The listing builds one solid part. Answer for the finished solid, in the listing's coordinates (mm). Face numbers are marked on the shaded views. A direction names the side the tool comes from. Round coordinates to 2 decimals unless told otherwise and drop trailing zeros. Order: outer loops, then holes, each group sorted by start corner. A loop starts at its lowest first (then second) coordinate and runs counter-clockwise, first axis right, second up. Notation, with made-up numbers: (18.5, 34.5) -> (57.5, 34.5) arc R19 cw to (57.5, 56.5) -> close; hole circle Ø3 at (8.25, 67). An arc over 180 degrees is marked (long way). Answer in a Markdown table with one row per item. Add a question column.
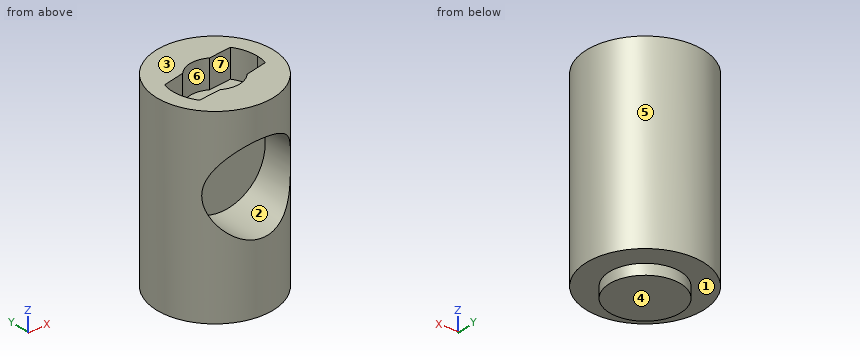
```python
from build123d import *

# Parameters (mm, degrees)
SKETCH_1_R          = 8.2
EXTRUDE_1_DEPTH     = 26.65
SKETCH_3_R          = 5
EXTRUDE_2_DEPTH     = 1.5
CUT_EXTRUDE_1_DEPTH = 4
CUT_EXTRUDE_START   = -1
SKETCH_5_R          = 6.25
CUT_EXTRUDE_2_DEPTH = 10


with BuildPart() as part:
    # Эскиз1 → Бобышка-Вытянуть1 (new body)
    with BuildSketch(Plane.XY):
        Circle(SKETCH_1_R)
    extrude(amount=EXTRUDE_1_DEPTH)

    # Эскиз3 → Бобышка-Вытянуть2 (add)
    with BuildSketch(Plane(origin=(0, 0, 0), x_dir=(-1, 0, 0), z_dir=(0, 0, -1))):
        Circle(SKETCH_3_R)
    extrude(amount=EXTRUDE_2_DEPTH)

    # Эскиз4 → Вырез-Вытянуть1 (cut)
    with BuildSketch(Plane.XY.offset(26.65)):
        with BuildLine():
            ThreePointArc((1.764967336, 3.022398105), (-0.563166375, 3.454394829), (-2.63353871, 2.305314265))
            Line((-2.63353871, 2.305314265), (-5.778686809, 1.614552185))
            ThreePointArc((-5.778686809, 1.614552185), (-5.921819707, -0.965428072), (-4.966654884, -3.366354001))
            Line((-4.966654884, -3.366354001), (-1.764967336, -3.022398105))
            ThreePointArc((-1.764967336, -3.022398105), (0.563166375, -3.454394829), (2.63353871, -2.305314265))
            Line((2.63353871, -2.305314265), (5.778686809, -1.614552185))
            ThreePointArc((5.778686809, -1.614552185), (5.944414221, -0.814824872), (6, 0))
            ThreePointArc((6, 0), (5.735849079, 1.760691724), (4.966654884, 3.366354001))
            Line((4.966654884, 3.366354001), (1.764967336, 3.022398105))
        make_face()
    extrude(amount=-CUT_EXTRUDE_1_DEPTH, mode=Mode.SUBTRACT)

    # Эскиз5 → Вырез-Вытянуть2 (cut)
    with BuildSketch(Plane(origin=(0, 0, 0), x_dir=(1, 0, 0), z_dir=(0, 1, 0)).offset(CUT_EXTRUDE_START)):
        with Locations((0, -16)):
            Circle(SKETCH_5_R)
    extrude(amount=-CUT_EXTRUDE_2_DEPTH, mode=Mode.SUBTRACT)


solid = part.part
```
1. The part is cut by section C-C (y = -4.5). Give the vertices of the cut face in (x, z).
2. The mould has two halves that part along Y. Classify the marked faces 4, 5, 6 and 7: released by +Y, released by -Y, zero draft, split by the parting line, or undercut.
3. The part is cut by section B-B (x = 0). Give the vertices of the cut face in (y, z).
4. For the marked faces 1, 2 and 3, determine the directions among +Z, -Z, +X, -X, +Y, -Y from which every point of the face is accessible in a straight line to the end or side of a thin tool.
5. Each of these flat-tipped pins is pushed along its axis until it touches: pin 1 (1 mm diameter, centred on x = 6.5, y = 6, fed in from +Z); pin 2 (2 mm diameter, centred on y = -2.5, z = 4.5, fed in from -X); pin 3 (1 mm diameter, centred on x = 2.5, z = 22, fed in from +Y). Where does it stop, or does it pass through?
6. The part is cut by section A-A (y = -6.25). Give the vertices of the cut face in (x, z).
7. The part is cut by section D-D (z = 11.5). Give the vertices of the cut face in (x, y).
8. Straight lines are drawn through the part: line 1 along Z through (x, y) = (0, -6.25); line 2 along Z through (x, y) = (0, -3); line 3 along X through (y, z) = (-4.25, 16). For each, find the intervals that lie inside material, in ascending order.
Report:
| question | item | result |
|---|---|---|
| 1 | outline | (-6.85, 0) -> (-2.18, 0) -> (-2.18, -1.5) -> (2.18, -1.5) -> (2.18, 0) -> (6.85, 0) -> (6.85, 26.65) -> (-6.85, 26.65) -> close; hole circle Ø12.5 at (0, 16) |
| 2 | face 4 | zero draft |
| 2 | face 5 | split by the parting line |
| 2 | face 6 | undercut |
| 2 | face 7 | undercut |
| 3 | outline | (-8.2, 0) -> (-5, 0) -> (-5, -1.5) -> (5, -1.5) -> (5, 0) -> (8.2, 0) -> (8.2, 26.65) -> (3.5, 26.65) -> (3.5, 22.65) -> (-3.5, 22.65) -> (-3.5, 26.65) -> (-8.2, 26.65) -> (-8.2, 22.25) -> (-1, 22.25) -> (-1, 9.75) -> (-8.2, 9.75) -> close |
| 4 | face 1 | -Z |
| 4 | face 2 | -Y |
| 4 | face 3 | +Z, +X, -X, +Y, -Y |
| 5 | pin 1 | passes through |
| 5 | pin 2 | stops at x = -8.06 |
| 5 | pin 3 | stops at y = 7.95 |
| 6 | outline | (-5.31, 0) -> (5.31, 0) -> (5.31, 12.7) arc R6.25 cw to (-5.31, 12.7) -> close; (-5.31, 19.3) arc R6.25 cw to (5.31, 19.3) -> (5.31, 26.65) -> (-5.31, 26.65) -> close |
| 7 | outline | (-4.34, -6.96) -> (-4.34, -1) -> (4.34, -1) -> (4.34, -6.96) arc R8.2 ccw (long way) to start |
| 8 | line 1 | z = 0 to 9.75, 22.25 to 26.65 |
| 8 | line 2 | z = -1.5 to 9.75, 22.25 to 22.65 |
| 8 | line 3 | x = -7.01 to -6.25, 6.25 to 7.01 |
